Input: dimensioned drawing with shaded views. Units: mm. Origin: part minimum x, y, z. Round coordinates to 2 decimals unless told otherwise and drop trailing zeros. Order: outer loops, then holes, each group sorted by start corner. A loop starts at its lowest first (then second) coordinate and runs counter-clockwise, first axis right, second up. Notation, with made-up numbers: M 45.5,-9 L 76.5,-9 A19 ccw 76.5,-2 Z; hole C -6.75,-30.5 d6. An arc over 180 degrees is marked long. Answer as CSV lines item,"result". Start each with the question number.
Item 1: Pull-direction query (X, two-part tool) for the marked faces 1 and 2; classes: +X half, -X half, draft (parallel to the pull), parting line (faces both ways), or undercut.
Item 2: Section query D-D on x = 31. Return the cut outline in (y, z), plus the area to 3 significant figures.
Item 3: Line query: line 1 (X direction, y = 30, z = 20); line 2 (Z direction, x = 9.5, y = 8); line 3 (X direction, y = 39, z = 6). Output: solid intervals per line, ascending. Write a range as [from, to].
Item 4: Section query C-C on y = 30. Return the cut outline in (x, z), plus the area to 3 significant figures.
Item 5: Section query A-A on x = 12. Return the cut outline in (y, z), plus the area to 3 significant figures.
Item 6: First-contact query: P1, Ø11, axis at x = 24.5, z = 18, coming from the +Y side; P2, Ø1.6, axis at y = 1.5, z = 19.5, coming from the -X side; P3, Ø6, axis at y = 25.5, z = 29, coming from the +X side. Flat tips, straight axial feed; report the tip coordinate or a pass-through.
Item 7: Section query B-B on z = 16.5. Return the cut outline in (x, y).
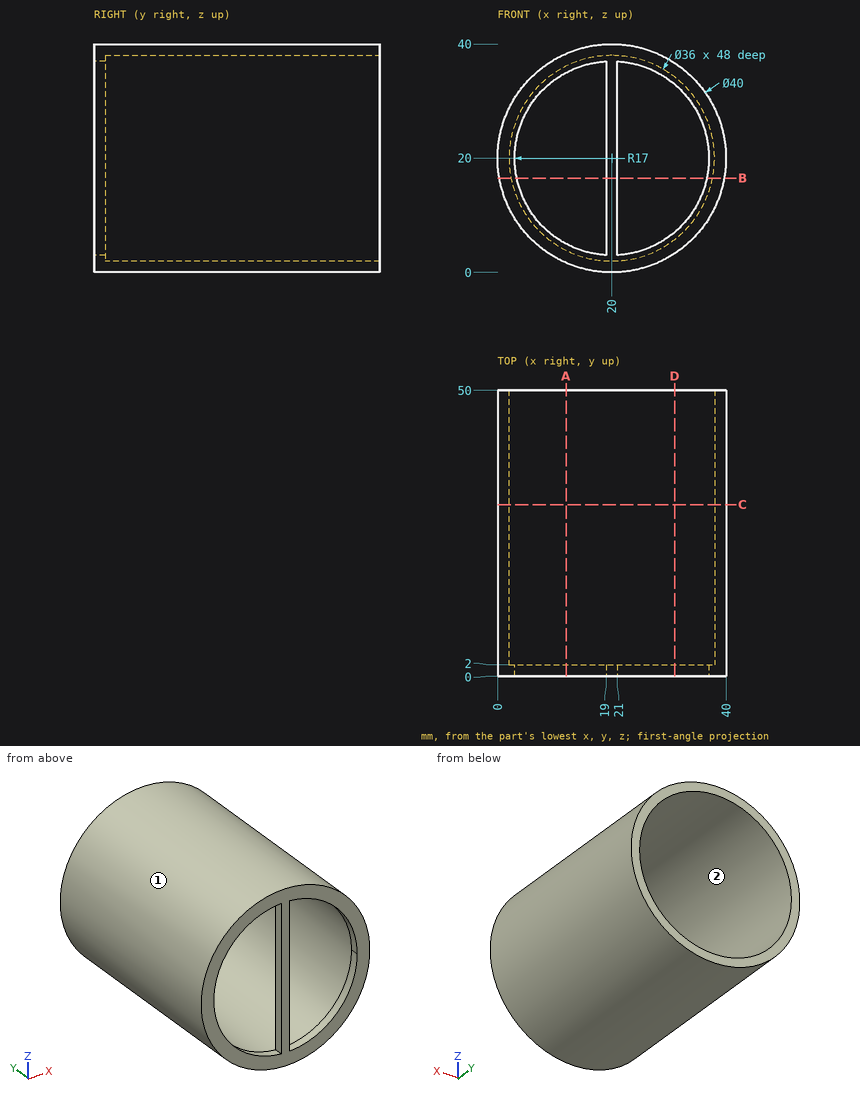
Results:
1,face 1,"parting line"
1,face 2,"undercut"
2,outline,"M 0,3.3 L 50,3.3 L 50,5.75 L 2,5.75 L 2,7.04 L 0,7.04 Z; M 0,32.96 L 2,32.96 L 2,34.25 L 50,34.25 L 50,36.7 L 0,36.7 Z"
2,area,"251 mm^2"
3,line 1,"[0, 2], [38, 40]"
3,line 2,"[2.98, 5.38], [34.62, 37.02]"
3,line 3,"[5.72, 8.69], [31.31, 34.28]"
4,outline,"C 20,20 d40; hole C 20,20 d36"
4,area,"239 mm^2"
5,outline,"M 0,1.67 L 50,1.67 L 50,3.88 L 2,3.88 L 2,5 L 0,5 Z; M 0,35 L 2,35 L 2,36.12 L 50,36.12 L 50,38.33 L 0,38.33 Z"
5,area,"225 mm^2"
6,P1,"y = 2"
6,P2,"x = 0"
6,P3,"x = 39.08"
7,outline,"M 0.31,0 L 3.36,0 L 3.36,2 L 2.34,2 L 2.34,50 L 0.31,50 Z; M 19,0 L 21,0 L 21,2 L 19,2 Z; M 36.64,0 L 39.69,0 L 39.69,50 L 37.66,50 L 37.66,2 L 36.64,2 Z"
